Autodesk Inventor part; units mm, degrees
ref_plane "YZ Plane" through (0, 0, 0) normal (1, 0, 0) x (0, 1, 0)
ref_plane "XZ Plane" through (0, 0, 0) normal (0, 1, 0) x (-1, 0, 0)
ref_plane "XY Plane" through (0, 0, 0) normal (0, 0, 1) x (1, 0, 0)
sketch "Sketch1" plane through (0, 0, 0) normal (0, 0, 1) x (1, 0, 0)
  circle A0 centre (0, 0) radius 3.25
  dimension "d0" = 6.5
extrude "Extrusion1" add sketch "Sketch1" along normal mid plane 14
sketch "Sketch2" plane through (0, 0, 7) normal (0, 0, 1) x (1, 0, 0)
  arc A0 (1.3601, -1.6) -> (-1.3601, -1.6) centre (0, 0) ccw
  line L0 (-1.3601, -1.6) -> (1.3601, -1.6)
  point P0 (0, 2.2)
  point P1 (0, -1.65)
  point P2 (0, -1.6)
  point P3 (0, 2.1)
  dimension "d4" = 2.1
  dimension "d12" = 3.7
extrude "Extrusion2" cut sketch "Sketch2" against normal blind 8.5
sketch "Sketch3" plane through (0, 0, -7) normal (0, 0, -1) x (-1, 0, 0)
  circle A0 centre (0, 0) radius 2.45
  dimension "d9" = 4.9
extrude "Extrusion3" add sketch "Sketch3" along normal blind 39.3
sketch "Sketch4" plane through (0, 0, -46.3) normal (0, 0, -1) x (-1, 0, 0)
  circle A0 centre (0, 0) radius 2.45
  arc A1 (-2.0106, 1.4) -> (-2.0106, -1.4) centre (0, 0) ccw
  arc A2 (2.0106, -1.4) -> (2.0106, 1.4) centre (0, 0) ccw
  line L0 (-2.0106, 1.4) -> (2.0106, 1.4)
  line L1 (2.0106, -1.4) -> (-2.0106, -1.4)
  dimension "d13" = 1.4
extrude "Extrusion4" add sketch "Sketch4" along normal blind 20 contours A0 L1 L0
properties part number "13042026-08"
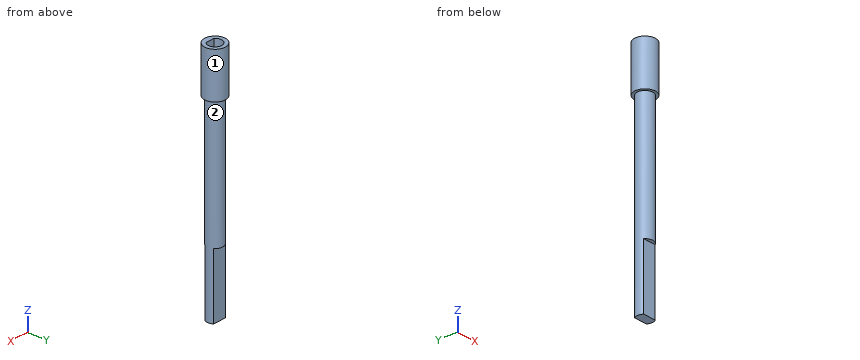
Source: CAD feature listing. Evaluate the final solid. Frame: model axes, mm. Face numbers are marked on the shaded views. A direction names the side the tool comes from. Round coordinates to 2 decimals unless told otherwise and drop trailing zeros. Loops run counter-clockwise (first coordinate to the right, second up) from the corner with the lowest first, then second, coordinate; pieces in that order, holes last.
Q1. Section A-A, the plane x = 0. Return loops of the section in (y, z).
Q2. Section D-D, the plane z = -4. Return loops of the section in (x, y).
Q3. Access query for the marked faces 1 and 2. Directions: +Z, -Z, +X, -X, +Y, -Y. A direction counts if a zero-diameter tool reaches every point of the face in a straight line with its end or side. Return the directions, or none.
Q4. Section C-C, the plane z = -18.5. Return loops of the section in (x, y), plus the area to 3 significant figures.
Q5. Ray query, line 1 (Y direction, x = 0, z = 4.75); line 2 (Y direction, x = 0.25, z = -51.5); line 3 (Z direction, x = -0.5, y = -2). Return the intervals inside material, ascending.
Q6. First-contact query: P1, Ø1.1, axis at x = 0.5, y = -0.5, coming from the +Z side; P2, Ø0.8, axis at x = 0.5, y = -2, coming from the -Z side; P3, Ø2, axis at y = 2, z = -44.5, coming from the -X side; P4, Ø0.8, axis at x = -0.5, z = 1.5, coming from the +Y side. Flat tips, straight axial feed; report the tip coordinate or a pass-through.
Q7. Section B-B, the plane y = 0. Return loops of the section in (x, z), plus the area to 3 significant figures.
Solutions:
1. outline: (-3.25, -7) - (-2.45, -7) - (-2.45, -46.3) - (-1.4, -46.3) - (-1.4, -66.3) - (1.4, -66.3) - (1.4, -46.3) - (2.45, -46.3) - (2.45, -7) - (3.25, -7) - (3.25, 7) - (2.1, 7) - (2.1, -1.5) - (-1.6, -1.5) - (-1.6, 7) - (-3.25, 7) - close
2. outline: circle Ø6.5 at (0, 0)
3. face 1: +Z, -Z
3. face 2: -Z
4. outline: circle Ø4.9 at (0, 0)
4. area: 18.9 mm2
5. line 1: y = -3.25 to -1.6, 2.1 to 3.25
5. line 2: y = -1.4 to 1.4
5. line 3: z = -46.3 to 7
6. P1: stops at z = -1.5
6. P2: stops at z = -46.3
6. P3: stops at x = -2.24
6. P4: stops at y = 3.25
7. outline: (-3.25, -7) - (-2.45, -7) - (-2.45, -66.3) - (2.45, -66.3) - (2.45, -7) - (3.25, -7) - (3.25, 7) - (2.1, 7) - (2.1, -1.5) - (-2.1, -1.5) - (-2.1, 7) - (-3.25, 7) - close
7. area: 346 mm2
